Build history of the part. All positions in model axes, mm. A direction names the side the tool comes from. Coordinates: 2 decimals unless noted, no trailing zeros. Loops run counter-clockwise (first coordinate to the right, second up) from the corner with the lowest first, then second, coordinate; pieces in that order, holes last. Notation, with made-up numbers: (-5, -3.5) -> (18, -3.5) arc R11 ccw to (18, 16.5) -> close; hole circle Ø4 at (82.5, 35.5). An arc over 180 degrees is marked (long way). One line per item, written item: value. Start each with the question number.
```python
from build123d import *

# Parameters (mm, degrees)
PAD002_DEPTH    = 18.5
THICKNESS001_T  = -1.5
PAD003_DEPTH    = 35
POCKET001_DEPTH = 35
SKETCH006_R     = 2
PAD004_DEPTH    = 10


with BuildPart() as part:
    # Sketch003 → Pad002 (new body)
    with BuildSketch(Plane.XY):
        Polygon((-6.7, -6.381475), (-6.7, -46.931937), (6.7, -46.931937), (6.7, -11.931937), (11.931937, -6.7), (46.931937, -6.7), (46.931937, 6.7), (6.381475, 6.7), align=None)
    extrude(amount=PAD002_DEPTH)

    # Thickness001
    thickness001_openings = [part.faces().sort_by_distance(p)[0] for p in [
        (0, -46.931937, 9.25),
        (46.931937, 0, 9.25),
    ]]
    offset(amount=THICKNESS001_T, openings=thickness001_openings)

    # Sketch004 (on Face8 of Thickness001) → Pad003 (join)
    with BuildSketch(Plane.XY.offset(18.5)):
        Polygon((-6.7, -6.381475), (6.381475, 6.7), (15.856706, -2.775231), (2.775231, -15.856706), align=None)
    extrude(amount=PAD003_DEPTH)

    # Sketch005 (on Face22 of Pad003) → Pocket001 (cut)
    with BuildSketch(Plane.XY.offset(53.5)):
        Polygon((-4.58, -6.381475), (6.381475, 4.58), (13.736706, -2.775231), (2.775231, -13.736706), align=None)
    extrude(amount=-POCKET001_DEPTH, mode=Mode.SUBTRACT)

    # Sketch006 (on Face4 of Pocket001) → Pad004 (join)
    with BuildSketch(Plane(origin=(0, 0, 0), x_dir=(1, 0, 0), z_dir=(0, 0, -1))):
        Polygon((6.7, 46.931937), (6.7, 11.931937), (11.931937, 6.7), (46.931937, 6.7), (46.931937, 46.931937), align=None)
        with Locations((17.80125, 17.80125)):
            Circle(SKETCH006_R, mode=Mode.SUBTRACT)
        with Locations((38.446656, 38.446656)):
            Circle(SKETCH006_R, mode=Mode.SUBTRACT)
    extrude(amount=-PAD004_DEPTH)


solid = part.part
```
Item 1: Band-saw the part on B-B, the plane z = 42. List the corners of the cut face in (x, y), and give its area (3 significant figures).
Item 2: Tool access for faces 1 (the face through (11.05, 2.03, 35.75)), 2 (the face through (29, -6.7, 14)), 3 (the face through (5, -4, 18.5)): list every direction of +Z, -Z, +X, -X, +Y, -Y with a clear straight run to the whole face (end or side of a thin tool).
Item 3: Band-saw the part on A-A, the plane y = -30. List the corners of the cut face in (x, z).
Item 4: Band-saw the part on D-D, the plane z = 5. List the corners of the cut face in (x, y).
Item 5: Two-plate mould, pull along Z, no slides. Class faces 4 (the face through (46.932, -26, 5)), 5 (the face through (-5.2, -27, 9)), 6 (the face through (0, -31, 18.5)): +Z half, -Z half, draft (parallel to the pull), parting line (faces both ways), or undercut.
Item 6: Drop flat-ended pins along their axis: pin 1 Ø5 at (x, y) = (38.45, -38.45) entering from +Z; pin 2 Ø6.5 at (x, y) = (-1, -21) entering from +Z; pin 3 Ø2.5 at (y, z) = (-30, 15) entering from +X. Give the stop position or say it passes through.
Item 7: Band-saw the part on C-C, the plane x = 26. List the corners of the cut face in (y, z), and give its area (3 significant figures).
Item 8: Probe probe 1 along X at (y, z) = (-38.5, 6); probe 2 along Z at (x, y) = (21, -1); probe 3 along X at (y, z) = (-12.5, 3). List the from-to ranges inside material, lowest first.
Worked out:
1. outline: (-6.7, -6.38) -> (2.78, -15.86) -> (15.86, -2.78) -> (6.38, 6.7) -> close; hole (-4.58, -6.38) -> (2.78, -13.74) -> (13.74, -2.78) -> (6.38, 4.58) -> close
1. area: 86.7 mm²
2. face 1: +Z, +X, +Y
2. face 2: +Z, +X, -Y
2. face 3: +Z
3. outline: (-6.7, 0) -> (46.93, 0) -> (46.93, 10) -> (6.7, 10) -> (6.7, 18.5) -> (-6.7, 18.5) -> close; hole (-5.2, 1.5) -> (5.2, 1.5) -> (5.2, 17) -> (-5.2, 17) -> close
4. outline: (-6.7, -46.93) -> (-5.2, -46.93) -> (-5.2, -7) -> (7, 5.2) -> (46.93, 5.2) -> (46.93, 6.7) -> (6.38, 6.7) -> (-6.7, -6.38) -> close; (5.2, -46.93) -> (46.93, -46.93) -> (46.93, -5.2) -> (11.93, -5.2) arc R1.5 ccw to (10.87, -5.64) -> (5.64, -10.87) arc R1.5 ccw to (5.2, -11.93) -> close; hole circle Ø4 at (17.8, -17.8); hole circle Ø4 at (38.45, -38.45)
5. face 4: draft
5. face 5: undercut
5. face 6: +Z half
6. pin 1: stops at z = 10
6. pin 2: stops at z = 18.5
6. pin 3: stops at x = 6.7
7. outline: (-46.93, 0) -> (6.7, 0) -> (6.7, 18.5) -> (-6.7, 18.5) -> (-6.7, 10) -> (-46.93, 10) -> close; hole (-5.2, 1.5) -> (5.2, 1.5) -> (5.2, 17) -> (-5.2, 17) -> close
7. area: 489 mm²
8. probe 1: x = -6.7 to -5.2, 5.2 to 36.45, 40.45 to 46.93
8. probe 2: z = 0 to 1.5, 17 to 18.5
8. probe 3: x = -6.7 to -5.2, 5.2 to 46.93
